Model file for the job. Use its own axes, mm. Face numbers are marked on the shaded views. A direction names the side the tool comes from. Give positions to 0.01 mm unless a question says otherwise; leave off trailing zeros. Write each loop counter-clockwise with the first axis right and the second up, starting at its lowest first coordinate (ties: lowest second). Pieces come first, ordered by that corner, then holes.
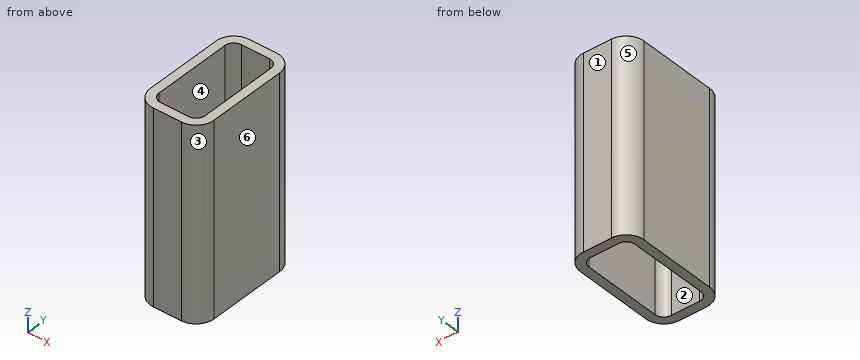
```python
from build123d import *

# Parameters (mm, degrees)
SKETCH_1_W      = 100
SKETCH_1_H      = 180
SKETCH_1_W_2    = 72
SKETCH_1_H_2    = 152
EXTRUDE_1_DEPTH = 300
FILLET_1_R      = 14
FILLET_2_R      = 28


with BuildPart() as part:
    # 草图1 → 凸台-拉伸1 (new body)
    with BuildSketch(Plane.XY):
        Rectangle(SKETCH_1_W, SKETCH_1_H)
        Rectangle(SKETCH_1_W_2, SKETCH_1_H_2, mode=Mode.SUBTRACT)
    extrude(amount=EXTRUDE_1_DEPTH)

    # 圆角1
    fillet_1_edges = [part.edges().sort_by_distance(p)[0] for p in [
        (-36, 76, 150),
        (-36, -76, 150),
        (36, -76, 150),
        (36, 76, 150),
    ]]
    fillet(fillet_1_edges, radius=FILLET_1_R)

    # 圆角2
    fillet_2_edges = [part.edges().sort_by_distance(p)[0] for p in [
        (-50, 90, 150),
        (50, 90, 150),
        (50, -90, 150),
        (-50, -90, 150),
    ]]
    fillet(fillet_2_edges, radius=FILLET_2_R)


solid = part.part
```
1. Pull direction Y, two halves, no side cores. Call the marked faces 3, 4, 5 and 6: +Y half, -Y half, draft (parallel to the pull), parting line (faces both ways), or undercut.
Calculated:
face 3: -Y half
face 4: undercut
face 5: +Y half
face 6: draft
2. Slice it at A-A, the plane y = -14. Write the cut outline in (x, z).
Calculated:
outline: (-50, 0) - (-36, 0) - (-36, 300) - (-50, 300) - close; (36, 0) - (50, 0) - (50, 300) - (36, 300) - close
3. Slice it at B-B, the plane x = 3.5. Write the cut outline in (y, z), and give its area (3 significant figures).
Calculated:
outline: (-90, 0) - (-76, 0) - (-76, 300) - (-90, 300) - close; (76, 0) - (90, 0) - (90, 300) - (76, 300) - close
area: 8,400 mm2
4. Slice it at C-C, the plane z = 260.5. Write the cut outline in (x, y), and give its area (3 significant figures).
Calculated:
outline: (-50, -62) arc R28 ccw to (-22, -90) - (22, -90) arc R28 ccw to (50, -62) - (50, 62) arc R28 ccw to (22, 90) - (-22, 90) arc R28 ccw to (-50, 62) - close; hole (-36, -62) arc R14 ccw to (-22, -76) - (22, -76) arc R14 ccw to (36, -62) - (36, 62) arc R14 ccw to (22, 76) - (-22, 76) arc R14 ccw to (-36, 62) - close
area: 6,550 mm2
5. Pin check, flat tips, straight feed: P1, Ø3, axis at x = 24, z = 190, coming from the +Y side; P2, Ø8, axis at x = 7.5, y = 69.5, coming from the +Z side. Stop position of each tip, or through.
Calculated:
P1: stops at y = 90
P2: passes through
6. Which spindle directions (+Z, -Z, +X, -X, +Y, -Y) get a long thin tool onto all of the face, cutting with end or side? Do the marked faces 1 and 2. Say none if no direction does.
Calculated:
face 1: +Z, -Z, +X, -X, +Y
face 2: +Z, -Z
7. Slice it at D-D, the plane x = 42. Write the cut outline in (y, z).
Calculated:
outline: (-81.6, 0) - (81.6, 0) - (81.6, 300) - (-81.6, 300) - close
8. Probe probe 1 along X at (y, z) = (-55, 30); probe 2 along Y at (x, z) = (-6.5, 255.5); probe 3 along Y at (x, z) = (-34, 17.5). List the from-to ranges inside material, lowest first.
Calculated:
probe 1: x = -50 to -36, 36 to 50
probe 2: y = -90 to -76, 76 to 90
probe 3: y = -87.3 to -69.21, 69.21 to 87.3
